from build123d import *

# Parameters (mm, degrees)
SKETCH_1_R      = 0.8
EXTRUDE_1_DEPTH = 1.6


with BuildPart() as part:
    # 스케치1 → 돌출1 (new body)
    with BuildSketch(Plane.XY):
        with BuildLine():
            Line((39, 0), (9, 0))
            ThreePointArc((9, 0), (2.268662967, 24.090162586), (0, 49))
            Line((0, 49), (14.5, 49))
            Line((14.5, 49), (14.5, 64.5))
            Line((14.5, 64.5), (47, 64.5))
            Line((47, 64.5), (47, 75.5))
            Line((47, 75.5), (14.5, 75.5))
            Line((14.5, 75.5), (14.5, 71))
            Line((14.5, 71), (0, 71))
            Line((0, 71), (0, 91))
            ThreePointArc((0, 91), (6.778150978, 109.821530225), (24, 120))
            Line((24, 120), (39, 120))
            Line((39, 120), (54, 120))
            ThreePointArc((54, 120), (71.221849022, 109.821530225), (78, 91))
            Line((78, 91), (78, 71))
            Line((78, 71), (63.5, 71))
            Line((63.5, 71), (63.5, 55.5))
            Line((63.5, 55.5), (31, 55.5))
            Line((31, 55.5), (31, 44.5))
            Line((31, 44.5), (63.5, 44.5))
            Line((63.5, 44.5), (63.5, 49))
            Line((63.5, 49), (78, 49))
            ThreePointArc((78, 49), (75.731337033, 24.090162586), (69, 0))
            Line((69, 0), (39, 0))
        make_face()
        with Locations((67, 75.5)):
            Circle(SKETCH_1_R, mode=Mode.SUBTRACT)
        with Locations((67, 44.5)):
            Circle(SKETCH_1_R, mode=Mode.SUBTRACT)
        with Locations(Location((11, 44.5, 0), (0, 0, 180))):
            Circle(SKETCH_1_R, mode=Mode.SUBTRACT)
        with Locations(Location((11, 75.5, 0), (0, 0, 180))):
            Circle(SKETCH_1_R, mode=Mode.SUBTRACT)
        with Locations(Location((4.25, 88, 0), (0, 0, 180))):
            Circle(SKETCH_1_R, mode=Mode.SUBTRACT)
        with Locations(Location((73.75, 88, 0), (0, 0, 180))):
            Circle(SKETCH_1_R, mode=Mode.SUBTRACT)
        with Locations(Location((18, 105, 0), (0, 0, 180))):
            Circle(SKETCH_1_R, mode=Mode.SUBTRACT)
        with Locations(Location((60, 105, 0), (0, 0, 180))):
            Circle(SKETCH_1_R, mode=Mode.SUBTRACT)
        with Locations(Location((26, 112, 0), (0, 0, 180))):
            Circle(SKETCH_1_R, mode=Mode.SUBTRACT)
        with Locations(Location((52, 112, 0), (0, 0, 180))):
            Circle(SKETCH_1_R, mode=Mode.SUBTRACT)
    extrude(amount=EXTRUDE_1_DEPTH)


solid = part.part
Input: part model. Units: mm. Frame: model coordinates. Round coordinates to 2 decimals unless told otherwise and drop trailing zeros. Write each loop counter-clockwise with the first axis right and the second up, starting at its lowest first coordinate (ties: lowest second). Pieces come first, ordered by that corner, then holes.
1) Cut plane C-C (y = 61). Return the cut outline in (x, z), then the cut area to 3 significant figures.
2) Ray query, L1, parallel to Y at x = 37, z = 0.25; L2, parallel to X at y = 112, z = 0.85; L3, parallel to X at y = 105, z = 1. Return the intervals inside material, ascending.
3) Cut plane D-D (y = 97.5). Return the cut outline in (x, z).
4) Cut plane B-B (z = 0.7). Count the separate pieces of the cut face and the enclosed holes in it, then the cut area to 3 significant figures.
5) Contact query for flat-ended pins moving along their axis: P1, Ø8, axis at x = 50.5, y = 89, coming from the -Z side; P2, Ø0.8, axis at y = 62, z = 0.5, coming from the +X side. Output: stop coordinate, or through.
6) Cut plane A-A (x = 29). Return the cut outline in (y, z), then the cut area to 3 significant figures.
Geometry says:
1. outline: (14.5, 0) - (63.5, 0) - (63.5, 1.6) - (14.5, 1.6) - close
1. area: 78.4 mm2
2. L1: y = 0 to 44.5, 55.5 to 64.5, 75.5 to 120
2. L2: x = 8.77 to 25.2, 26.8 to 51.2, 52.8 to 69.23
2. L3: x = 3.53 to 17.2, 18.8 to 59.2, 60.8 to 74.47
3. outline: (0.72, 0) - (77.28, 0) - (77.28, 1.6) - (0.72, 1.6) - close
4. separate pieces: 1
4. enclosed holes: 10
4. area: 7,350 mm2
5. P1: stops at z = 0
5. P2: stops at x = 63.5
6. outline: (0, 0) - (64.5, 0) - (64.5, 1.6) - (0, 1.6) - close; (75.5, 0) - (120, 0) - (120, 1.6) - (75.5, 1.6) - close
6. area: 174 mm2
